Geometry check sheet. Reference: the model listing, model coordinates, mm. Face numbers are marked on the shaded views. A direction names the side the tool comes from. Give positions to 0.01 mm unless a question says otherwise; leave off trailing zeros.
1. Go/stop test with flat-tipped pins: pin 1 Ø6 at (x, z) = (22.5, 8) entering from -Y; pin 2 Ø2.5 at (x, y) = (2.5, -25) entering from -Z; pin 3 Ø15 at (x, y) = (26, 10) entering from +Z. Record where each tip stops, or that it passes through.
2. Material ranges on L1, parallel to X at y = 17, z = 4.5; L2, parallel to Y at x = 23, z = -5; L3, parallel to X at y = -19, z = -3.5, recorded low to high.
3. Release check for a two-part mould opening along Y. For the marked faces 1, 2, 3 and 4 record: +Y half, -Y half, draft (parallel to the pull), parting line (faces both ways), or undercut.
4. Tool access check on the marked faces 5 and 6. Record the directions out of +Z, -Z, +X, -X, +Y, -Y that give a thin tool (end or side, any length) a straight path to the whole face; none if there is none.
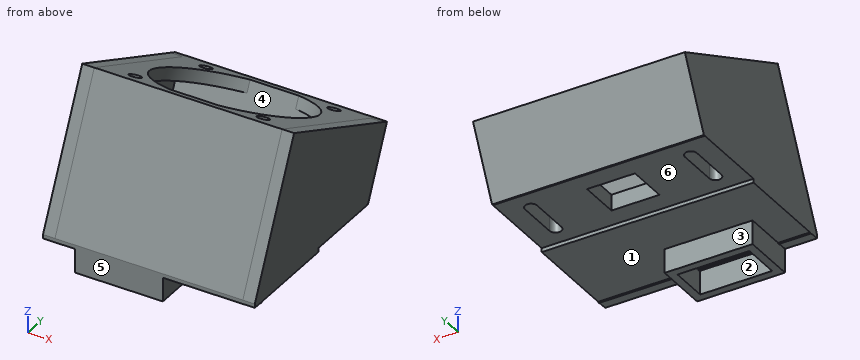
from build123d import *

# Parameters (mm, degrees)
SKETCH_W      = 53
SKETCH_H      = 20
SKETCH_W_2    = 12
SKETCH_H_2    = 10
PAD_DEPTH     = 4
PAD001_DEPTH  = 3
PAD002_DEPTH  = 3
SKETCH002_W   = 53
SKETCH002_H   = 38.0651251893
PAD003_DEPTH  = 3
SKETCH003_W   = 53
SKETCH003_H   = 42
SKETCH003_R   = 19
SKETCH003_R_2 = 1.5
PAD004_DEPTH  = 3
SKETCH004_W   = 53
SKETCH004_H   = 18.48
PAD005_DEPTH  = 3
SKETCH005_W   = 53
SKETCH005_H   = 26
SKETCH005_W_2 = 18
SKETCH005_H_2 = 8
PAD006_DEPTH  = 1
SKETCH006_W   = 22
SKETCH006_H   = 13.310112688
SKETCH006_W_2 = 18
SKETCH006_H_2 = 9.310112688
PAD007_DEPTH  = 6


with BuildPart() as part:
    # Sketch → Pad (new body)
    with BuildSketch(Plane.XY):
        with Locations((26.5, 10)):
            Rectangle(SKETCH_W, SKETCH_H)
        with BuildLine():
            ThreePointArc((48, 15), (46.5, 16.5), (45, 15))
            Line((45, 15), (45, 5))
            ThreePointArc((45, 5), (46.5, 3.5), (48, 5))
            Line((48, 15), (48, 5))
        make_face(mode=Mode.SUBTRACT)
        with BuildLine():
            ThreePointArc((8, 15), (6.5, 16.5), (5, 15))
            Line((5, 15), (5, 5))
            ThreePointArc((5, 5), (6.5, 3.5), (8, 5))
            Line((8, 15), (8, 5))
        make_face(mode=Mode.SUBTRACT)
        with Locations((26.5, 10)):
            Rectangle(SKETCH_W_2, SKETCH_H_2, mode=Mode.SUBTRACT)
    extrude(amount=PAD_DEPTH)

    # Sketch001 (on Face1 of Pad) → Pad001 (join)
    with BuildSketch(Plane(origin=(0, 0, 0), x_dir=(0, -1, 0), z_dir=(-1, 0, 0))):
        Polygon((-26.3390883587, 17.5947033355), (9.9134538694, 34.4989389586), (26, 0), (0, 0), (0, 4), (-20, 4), align=None)
    extrude(amount=-PAD001_DEPTH)

    # CopySketch002 → Pad002 (join)
    with BuildSketch(Plane(origin=(53, 0, 0), x_dir=(0, -1, 0), z_dir=(-1, 0, 0))):
        Polygon((-26.3390883587, 17.5947033355), (9.9134538694, 34.4989389586), (26, 0), (0, 0), (0, 4), (-20, 4), align=None)
    extrude(amount=PAD002_DEPTH)

    # Sketch002 (on Face30 of Pad002) → Pad003 (join)
    with BuildSketch(Plane(origin=(0, -21.3565107925, 9.9583496311), x_dir=(1, 0, 0), z_dir=(0, -0.9063135557, 0.4226058906))):
        with Locations((26.5, 8.0448094397)):
            Rectangle(SKETCH002_W, SKETCH002_H)
    extrude(amount=-PAD003_DEPTH)

    # Sketch003 (on Face27 of Pad003) → Pad004 (join)
    with BuildSketch(Plane(origin=(0, 11.4430569231, 24.5405893275), x_dir=(1, 0, 0), z_dir=(0, 0.4226058906, 0.9063135557))):
        with Locations((26.5, -2.5641524483)):
            Rectangle(SKETCH003_W, SKETCH003_H)
        with Locations((26.5, -2.5641524483)):
            Circle(SKETCH003_R, mode=Mode.SUBTRACT)
        with Locations((42.5, 13.4358475517)):
            Circle(SKETCH003_R_2, mode=Mode.SUBTRACT)
        with Locations((10.5, 13.4358475517)):
            Circle(SKETCH003_R_2, mode=Mode.SUBTRACT)
        with Locations((10.5, -18.5641524483)):
            Circle(SKETCH003_R_2, mode=Mode.SUBTRACT)
        with Locations((42.5, -18.5641524483)):
            Circle(SKETCH003_R_2, mode=Mode.SUBTRACT)
    extrude(amount=-PAD004_DEPTH)

    # Sketch004 (on Face41 of Pad004) → Pad005 (join)
    with BuildSketch(Plane(origin=(0, 16.708658547, -7.7910977731), x_dir=(-1, 0, 0), z_dir=(0, 0.9063135557, -0.4226058906))):
        with Locations((-26.5, 17.8373720343)):
            Rectangle(SKETCH004_W, SKETCH004_H)
    extrude(amount=-PAD005_DEPTH)

    # Sketch005 (on Face6 of Pad005) → Pad006 (join)
    with BuildSketch(Plane(origin=(0, 0, 0), x_dir=(1, 0, 0), z_dir=(0, 0, -1))):
        with Locations((26.5, 13)):
            Rectangle(SKETCH005_W, SKETCH005_H)
        with Locations((19, 18.689887312)):
            Rectangle(SKETCH005_W_2, SKETCH005_H_2, mode=Mode.SUBTRACT)
    extrude(amount=PAD006_DEPTH)

    # Sketch006 (on Face27 of Pad006) → Pad007 (join)
    with BuildSketch(Plane(origin=(0, 0, -1), x_dir=(1, 0, 0), z_dir=(0, 0, -1))):
        with Locations((19, 19.344943656)):
            Rectangle(SKETCH006_W, SKETCH006_H)
        with Locations((19, 19.344943656)):
            Rectangle(SKETCH006_W_2, SKETCH006_H_2, mode=Mode.SUBTRACT)
    extrude(amount=PAD007_DEPTH)


solid = part.part
Result:
1. pin 1: stops at y = -23.67
1. pin 2: stops at z = -1.05
1. pin 3: stops at z = 4
2. L1: x = 0 to 3, 50 to 53
2. L2: y = -26 to -24, -14.69 to -12.69
2. L3: x = 8 to 10, 28 to 30
3. face 1: draft
3. face 2: undercut
3. face 3: +Y half
3. face 4: undercut
4. face 5: +Z, -Z, +X, -X, -Y
4. face 6: -Z, +X, -X, +Y
